Part model, mm, in its own coordinate system. Face numbers are marked on the shaded views. Give positions to 0.01 mm unless a question says otherwise; leave off trailing zeros. Order: outer loops, then holes, each group sorted by start corner. A loop starts at its lowest first (then second) coordinate and runs counter-clockwise, first axis right, second up. Notation, with made-up numbers: (-39.5, 59.5) -> (-26.5, 59.5) arc R26 cw to (-26.5, 75.5) -> close; hole circle Ø10 at (38, -29). An arc over 180 degrees is marked (long way). Write item = value, one per line. Start each with the question number.
(1) Saw through at D-D, the plane z = 3. List the corners of the cut face in (x, y), then the cut area to 3 significant figures.
(2) Flat gauge pin, fed straight in: pin 1 (1 mm diameter, centred on x = -1.5, y = 1.5, fed in from -Z). Where does the tip first touch, or does it go through?
(3) Probe line 1 along Z through (x, y) = (-1.45, 1.95); line 2 along X through (y, z) = (0.55, -1); line 3 along Z through (x, y) = (-0.9, 0.9). List the from-to ranges inside material, lowest first. Write a range as from..to.
(4) Saw through at C-C, the plane y = 0.55. List the corners of the cut face in (x, z) (3 decimals).
(5) Saw through at A-A, the plane x = -1.4. List the corners of the cut face in (y, z).
(6) Saw through at B-B, the plane z = 0. List the corners of the cut face in (x, y), then the cut area to 3 significant figures.
(7) Two-plate mould, pull along Z, no slides. Class the marked faces 1, 2 and 3: pulls with the +Z half, pulls with the -Z half, needs draft (parallel to the pull), parting line crosses it, or undercut.
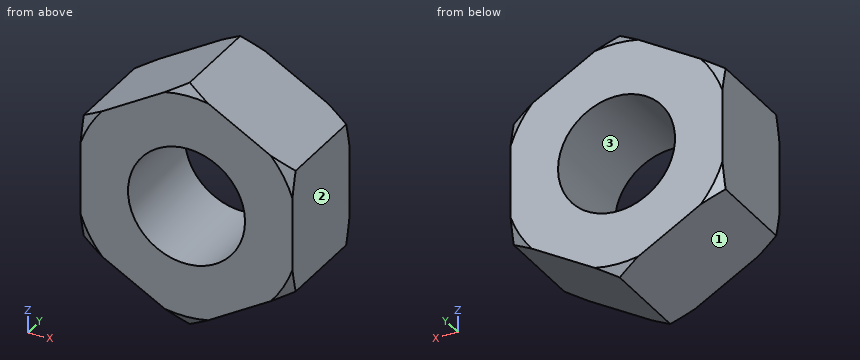
from build123d import *

# Parameters (mm, degrees)
SKETCH_1_R          = 3.85
EXTRUDE_1_DEPTH     = 3
CHAMFER_6_SIZE      = 0.4
CHAMFER_6_SIZE2     = 0.692820323
CHAMFER_7_SIZE      = 0.4
CHAMFER_7_SIZE2     = 0.692820323
SKETCH_3_OUTSIDE_W  = 11.96
SKETCH_3_OUTSIDE_H  = 11.96
CUT_EXTRUDE_4_DEPTH = 3
HOLE_WIZARD_M42_D   = 3.3


with BuildPart() as part:
    # Эскиз1 → Бобышка-Вытянуть1 (new body)
    with BuildSketch(Plane(origin=(0, 0, 0), x_dir=(1, 0, 0), z_dir=(0, 1, 0))):
        with Locations(Location((0, 0, 0), (0, 0, 270))):
            Circle(SKETCH_1_R)
    extrude(amount=EXTRUDE_1_DEPTH)

    # Фаска6
    chamfer_6_edges = [part.edges().sort_by_distance(p)[0] for p in [
        (0, 0, -3.85),
    ]]
    chamfer_6_side = [part.faces().sort_by_distance(p)[0] for p in [
        (0, 1.5, -3.85),
    ]]
    chamfer(chamfer_6_edges, length=CHAMFER_6_SIZE, length2=CHAMFER_6_SIZE2, reference=chamfer_6_side[0])

    # Фаска7
    chamfer_7_edges = [part.edges().sort_by_distance(p)[0] for p in [
        (0, 3, -3.85),
    ]]
    chamfer_7_side = [part.faces().sort_by_distance(p)[0] for p in [
        (0, 1.7, -3.85),
    ]]
    chamfer(chamfer_7_edges, length=CHAMFER_7_SIZE, length2=CHAMFER_7_SIZE2, reference=chamfer_7_side[0])

    # Эскиз3 outside → Вырез-Вытянуть4 (cut)
    with BuildSketch(Plane(origin=(0, 3, 0), x_dir=(1, 0, 0), z_dir=(0, 1, 0))):
        Rectangle(SKETCH_3_OUTSIDE_W, SKETCH_3_OUTSIDE_H)
        Polygon((2.987787643, -1.725), (2.987787643, 1.725), (0, 3.45), (-2.987787643, 1.725), (-2.987787643, -1.725), (0, -3.45), align=None, mode=Mode.SUBTRACT)
    extrude(amount=-CUT_EXTRUDE_4_DEPTH, mode=Mode.SUBTRACT)

    # Отверстие обработанное метчиком M42 (through all)
    with Locations(Plane(origin=(0, 0, 0), x_dir=(-1, 0, 0), z_dir=(0, -1, 0))):
        with Locations((0, 0)):
            Hole(HOLE_WIZARD_M42_D / 2)


solid = part.part
Results list:
q1.outline = (-0.78, 0) -> (0.78, 0) -> (0.78, 3) -> (-0.78, 3) -> close
q1.area = 4.68 mm^2
q2.pin_1 = -2.87
q3.line_1 = -2.61..-0.79, 0.79..2.61
q3.line_2 = -2.99..-1.31, 1.31..2.99
q3.line_3 = -2.93..-1.38, 1.38..2.93
q4.outline = (-2.988, -1.725) -> (0, -3.45) -> (2.988, -1.725) -> (2.988, 1.725) -> (0, 3.45) -> (-2.988, 1.725) -> close; hole circle Ø3.3 at (0, 0)
q5.outline = (0, -2.64) -> (3, -2.64) -> (3, -0.87) -> (0, -0.87) -> close; (0, 0.87) -> (3, 0.87) -> (3, 2.64) -> (0, 2.64) -> close
q6.outline = (-2.99, 0) -> (-1.65, 0) -> (-1.65, 3) -> (-2.99, 3) -> close; (1.65, 0) -> (2.99, 0) -> (2.99, 3) -> (1.65, 3) -> close
q6.area = 8.03 mm^2
q7.face_1 = pulls with the -Z half
q7.face_2 = needs draft
q7.face_3 = undercut
